from build123d import *

# Parameters (mm, degrees)
F0_W      = 576
F0_H      = 598
F1_DEPTH  = 50.1
F3_W      = 51
F3_H      = 51
F4_DEPTH  = 298.5
F8_DEPTH  = 5
F12_DEPTH = 5
F13_W     = 814
F13_H     = 60
F14_DEPTH = 5
F16_D     = 7
F18_D     = 7
F20_D     = 7
F20_DEPTH = 15
F20_TIP   = 2.1030121666
F23_D     = 6
F23_DEPTH = 15
F23_TIP   = 1.8025818571


with BuildPart() as f1:
    # F0 (on Front) → F1 (new body)
    with BuildSketch(Plane.XZ):
        Polygon((51, 0), (0, 0), (0, -51), (0, -649), (0, -700), (0, -1294), (51, -1294), (51, -700), (627, -700), (627, -1294), (678, -1294), (678, -700), (678, -649), (678, -51), (678, 0), (627, 0), align=None)
        with Locations((339, -350)):
            Rectangle(F0_W, F0_H, mode=Mode.SUBTRACT)
    extrude(amount=F1_DEPTH)

    # F3 (on face) → F4 (join)
    with BuildSketch(Plane(origin=(0, 0, 0), x_dir=(-1, 0, 0), z_dir=(0, 1, 0))):
        with Locations((-25.5, -25.5)):
            Rectangle(F3_W, F3_H)
        with Locations((-652.5, -25.5)):
            Rectangle(F3_W, F3_H)
        with Locations((-652.5, -674.5)):
            Rectangle(F3_W, F3_H)
        with Locations((-25.5, -674.5)):
            Rectangle(F3_W, F3_H)
    extrude(amount=F4_DEPTH)

    # F5: F1 across plane


with BuildPart() as f1_1:
    add(f1.part)
    add(f1.part.mirror(Plane.XZ.offset(-298.5)))

    # F7 (on offset) → F8 (join)
    with BuildSketch(Plane.XY.offset(-50.1)):
        Polygon((51, 0), (102, 0), (51, 51), align=None)
        Polygon((51, 597), (51, 546), (102, 597), align=None)
        Polygon((576, 597), (627, 546), (627, 597), align=None)
        Polygon((627, 0), (627, 51), (576, 0), align=None)
    extrude(amount=F8_DEPTH)

    # F10 (on offset) → F12 (join)
    with BuildSketch(Plane.YZ.offset(50.1)):
        Polygon((51, -51), (0, -51), (0, -102), align=None)
        Polygon((546, -51), (597, -102), (597, -51), align=None)
        Polygon((0, -649), (51, -649), (0, -598), align=None)
        Polygon((597, -598), (546, -649), (597, -649), align=None)
    extrude(amount=-F12_DEPTH)

    # F13 (on face) → F14 (join)
    with BuildSketch(Plane(origin=(0, 0, -1294), x_dir=(1, 0, 0), z_dir=(0, 0, -1))):
        with Locations((339, 25.5)):
            Rectangle(F13_W, F13_H)
        with Locations((339, -622.5)):
            Rectangle(F13_W, F13_H)
    extrude(amount=F14_DEPTH)

    # F16 (through all)
    with Locations(Plane.XY.offset(-45.1)):
        with Locations((66, 582), (612, 582), (612, 15), (66, 15)):
            Hole(F16_D / 2)

    # F18 (through all)
    with Locations(Plane.YZ.offset(50.1)):
        with Locations((15, -632.2), (582, -632.2), (582, -66), (15, -66)):
            Hole(F18_D / 2)

    # F20
    with Locations(Plane(origin=(0, 0, 0), x_dir=(0, -1, 0), z_dir=(-1, 0, 0))):
        with Locations((-612, -174.75), (-472.35, -36), (-124.65, -36), (15, -174.75), (15, -523.45), (-124.65, -662.2), (-472.35, -662.2), (-612, -523.45)):
            Hole(F20_D / 2, depth=F20_DEPTH)
            with Locations((0, 0, -(F20_DEPTH + F20_TIP / 2))):  # 118° drill point
                Cone(0, F20_D / 2, F20_TIP, mode=Mode.SUBTRACT)

    # F23
    with Locations(Plane.XY):
        with Locations((174.5, -15), (36, 124.4), (36, 472.6), (174.5, 612), (503.5, 612), (642, 472.6), (642, 124.4), (503.5, -15)):
            Hole(F23_D / 2, depth=F23_DEPTH)
            with Locations((0, 0, -(F23_DEPTH + F23_TIP / 2))):  # 118° drill point
                Cone(0, F23_D / 2, F23_TIP, mode=Mode.SUBTRACT)


solid = f1_1.part
Here's how the part is built. I have some questions about the finished solid (model axes, mm). A direction names the side the tool comes from. Coordinates: 2 decimals unless noted, no trailing zeros. Order: outer loops, then holes, each group sorted by start corner. A loop starts at its lowest first (then second) coordinate and runs counter-clockwise, first axis right, second up. Notation, with made-up numbers: (25.5, 38.5) -> (46.5, 38.5) arc R15 cw to (46.5, 48.5) -> close; hole circle Ø11 at (49, 4.5). An arc over 180 degrees is marked (long way). Answer in a Markdown table with one row per item.
(1) On a 3-axis mill with a long thin cutter (end or side, diameter ignored), from which of +Z, -Z, +X, -X, +Y, -Y can I reach the whole of each face in a straight line? I mean faces 4 (the face through (48, 572, -623)), 5 (the face through (653, 303, -700)), 6 (the face through (678, 297, -650)), 7 (the face through (45.1, 19, -70)). Say none if no direction works.
Answer key:
| item | result |
|---|---|
| face 4 | +X, -X |
| face 5 | -Z, +X, -X |
| face 6 | +Z, +X, +Y, -Y |
| face 7 | -X |
(2) Please list where these lines run through material, in increasing order: probe 1 along Z at (x, y) = (8.25, 612); probe 2 along Y at (x, z) = (174, -2); probe 3 along Y at (x, z) = (10.5, -36).
Answer key:
| item | result |
|---|---|
| probe 1 | -1299 to -526.95, -519.95 to -178.25, -171.25 to 0 |
| probe 2 | -50.1 to -17.96, -12.04 to 0, 597 to 609.04, 614.96 to 647.1 |
| probe 3 | -50.1 to 121.15, 128.15 to 468.85, 475.85 to 647.1 |
(3) Will these pins go through, and if not, where does the flat tip stop? pin 1 Ø7 at (x, y) = (503.5, -15) entering from +Z; pin 2 Ø1.5 at (x, z) = (632, -289.5) entering from +Y; pin 3 Ø6 at (x, z) = (42.5, -328.5) entering from -Y; pin 4 Ø11 at (y, z) = (612, -523.45) entering from +X.
Answer key:
| item | result |
|---|---|
| pin 1 | z = 0 |
| pin 2 | y = 647.1 |
| pin 3 | y = -50.1 |
| pin 4 | x = 678 |
(4) I want a section at C-C on x = 131. List the corners of the cut face in (y, z) for me, then the cut area to 3 significant figures.
Answer key:
| item | result |
|---|---|
| outline | (-55.5, -1299) -> (4.5, -1299) -> (4.5, -1294) -> (-55.5, -1294) -> close; (-50.1, -700) -> (0, -700) -> (0, -649) -> (-50.1, -649) -> close; (-50.1, -51) -> (0, -51) -> (0, 0) -> (-50.1, 0) -> close; (592.5, -1299) -> (652.5, -1299) -> (652.5, -1294) -> (592.5, -1294) -> close; (597, -700) -> (647.1, -700) -> (647.1, -649) -> (597, -649) -> close; (597, -51) -> (647.1, -51) -> (647.1, 0) -> (597, 0) -> close |
| area | 10,800 mm^2 |
(5) I want a section at A-A on z = -344.5. List the corners of the cut face in (x, y) for me, then the cut area to 3 significant figures.
Answer key:
| item | result |
|---|---|
| outline | (0, -50.1) -> (51, -50.1) -> (51, 0) -> (0, 0) -> close; (0, 597) -> (51, 597) -> (51, 647.1) -> (0, 647.1) -> close; (627, -50.1) -> (678, -50.1) -> (678, 0) -> (627, 0) -> close; (627, 597) -> (678, 597) -> (678, 647.1) -> (627, 647.1) -> close |
| area | 10,200 mm^2 |
(6) Thinking about a two-plate mould opening in X: for faces 1 (the face through (602, 26, -48)), 2 (the face through (50.1, 582, -70)), 3 (the face through (0, 300, -650)), which applies, +X half, -X half, draft (parallel to the pull), parting line (faces both ways), or undercut?
Answer key:
| item | result |
|---|---|
| face 1 | undercut |
| face 2 | +X half |
| face 3 | -X half |
(7) I want a section at B-B on y = 145.5. List the corners of the cut face in (x, z) for me, then the cut area to 3 significant figures.
Answer key:
| item | result |
|---|---|
| outline | (0, -700) -> (51, -700) -> (51, -649) -> (0, -649) -> close; (0, -51) -> (51, -51) -> (51, 0) -> (0, 0) -> close; (627, -700) -> (678, -700) -> (678, -649) -> (627, -649) -> close; (627, -51) -> (678, -51) -> (678, 0) -> (627, 0) -> close |
| area | 10,400 mm^2 |
